Verification items for the finished model (mm, model axes). A direction names the side the tool comes from. Give positions to 0.01 mm unless a question says otherwise; leave off trailing zeros. Loops run counter-clockwise (first coordinate to the right, second up) from the corner with the lowest first, then second, coordinate; pieces in that order, holes last. Notation, with made-up numbers: M -14,86.5 L 28,86.5 A35 cw 28,123.5 Z; hole C 44,-11.5 d11. An arc over 180 degrees is marked long. Use a Markdown table: item, result.
from build123d import *

# Parameters (mm, degrees)
SKETCH1_R           = 87.5
SKETCH1_R_2         = 70
BOSS_EXTRUDE1_DEPTH = 570
CHAMFER1_SIZE       = 5
SKETCH3_W           = 46
SKETCH3_H           = 23.271648671
CHAMFER2_SIZE       = 3
CHAMFER3_SIZE       = 2
SKETCH4_R           = 5
CUT_EXTRUDE1_DEPTH  = 102


with BuildPart() as part:
    # Sketch1 → Boss-Extrude1 (new body, symmetric)
    with BuildSketch(Plane.XY):
        Circle(SKETCH1_R)
        Circle(SKETCH1_R_2, mode=Mode.SUBTRACT)
    extrude(amount=BOSS_EXTRUDE1_DEPTH, both=True)

    # Chamfer1
    chamfer1_edges = [part.edges().sort_by_distance(p)[0] for p in [
        (-87.5, 0, -570),
    ]]
    chamfer(chamfer1_edges, length=CHAMFER1_SIZE)

    # Sketch3 → Cut-Revolve1 (revolve, cut)
    with BuildSketch(Plane(origin=(0, 0, 0), x_dir=(0, 0, -1), z_dir=(1, 0, 0))):
        with Locations((-547, 95.635824336)):
            Rectangle(SKETCH3_W, SKETCH3_H)
    revolve(axis=Axis((0, 0, 0), (0, 0, 1)), mode=Mode.SUBTRACT)

    # Chamfer2
    chamfer2_edges = [part.edges().sort_by_distance(p)[0] for p in [
        (0, -84, 570),
    ]]
    chamfer(chamfer2_edges, length=CHAMFER2_SIZE)

    # Chamfer3
    chamfer3_edges = [part.edges().sort_by_distance(p)[0] for p in [
        (-70, 0, 570),
    ]]
    chamfer(chamfer3_edges, length=CHAMFER3_SIZE)

    # Sketch4 → Cut-Extrude1 (cut)
    with BuildSketch(Plane(origin=(0, 0, 0), x_dir=(1, 0, 0), z_dir=(0, 1, 0))):
        with Locations((0, 540)):
            Circle(SKETCH4_R)
    extrude(amount=CUT_EXTRUDE1_DEPTH, mode=Mode.SUBTRACT)


solid = part.part
(1) Cross-section at B-B on z = 236. Record the cut outline in (x, y), then the cut area to 3 significant figures.
Results below:
| item | result |
|---|---|
| outline | C 0,0 d175; hole C 0,0 d140 |
| area | 8,660 mm^2 |
(2) Gauge pin test, flat ends, axial feed: P1, Ø12, axis at x = -27, z = 42.5, coming from the +Y side; P2, Ø1, axis at x = -37.5, z = 341.5, coming from the -Y side; P3, Ø6, axis at y = -67.5, z = 38.5, coming from the +X side. Record the tip position at first contact, or that the pin passes through.
Results below:
| item | result |
|---|---|
| P1 | y = 84.94 |
| P2 | y = -79.29 |
| P3 | x = 59.13 |
(3) Material ranges on line 1 (Y direction, x = 0, z = -232); line 2 (Z direction, x = 0, y = 77); line 3 (X direction, y = 21, z = -149.5), recorded low to high.
Results below:
| item | result |
|---|---|
| line 1 | -87.5 to -70, 70 to 87.5 |
| line 2 | -570 to -545, -535 to 570 |
| line 3 | -84.94 to -66.78, 66.78 to 84.94 |
(4) Draft check along Y on faces 1 (the flat face through (-37, -61, -570)), 2 (the cylindrical face through (-55.55, -42.594, -8.966)), 3 (the conical face through (-65.66, -50.35, -569.76)). Enter one of: +Y half, -Y half, draft (parallel to the pull), parting line (faces both ways), or undercut.
Results below:
| item | result |
|---|---|
| face 1 | draft |
| face 2 | undercut |
| face 3 | parting line |
(5) Cross-section at A-A on y = 0. Record the cut outline in (x, z), then the cut area to 3 significant figures.
Results below:
| item | result |
|---|---|
| outline | M -87.5,-565 L -82.5,-570 L -70,-570 L -70,568 L -72,570 L -81,570 L -84,567 L -84,524 L -87.5,524 Z; M 70,-570 L 82.5,-570 L 87.5,-565 L 87.5,524 L 84,524 L 84,567 L 81,570 L 72,570 L 70,568 Z |
| area | 39,500 mm^2 |
(6) Set-up check for faces 4 (the flat face through (-33, 78, 524)), 5 (the cylindrical face through (-64.49, 59.14, -12.88)): record each of +Z, -Z, +X, -X, +Y, -Y from which the full face is reachable in a straight line by a thin tool's end or side.
Results below:
| item | result |
|---|---|
| face 4 | +Z |
| face 5 | +Z, -Z |
